For this review, take the finished solid that the model builds, in its own axes (mm). A direction names the side the tool comes from. Round coordinates to 2 decimals unless told otherwise and drop trailing zeros. Order: outer loops, then holes, each group sorted by start corner. A loop starts at its lowest first (then second) coordinate and runs counter-clockwise, first axis right, second up. Notation, with made-up numbers: (80.25, 17) - (135.25, 17) arc R14 cw to (135.25, 41) - close; hole circle Ø3 at (-21, 44.25). An arc over 180 degrees is marked (long way). One line per question, with ' | ' between items.
```python
from build123d import *

# Parameters (mm, degrees)
F0_R     = 15.875
F1_DEPTH = 19.05
F2_R     = 1.27
F3_R     = 6.35
F4_DEPTH = 25.4
F5_R     = 3.175
F6_DEPTH = 12.7


with BuildPart() as f1:
    # F0 (on Front) → F1 (new body)
    with BuildSketch(Plane.XZ):
        Circle(F0_R)
    extrude(amount=-F1_DEPTH)

    # F2
    f2_edges = [f1.edges().sort_by_distance(p)[0] for p in [
        (-15.875, 19.05, 0),
        (-15.875, 0, 0),
    ]]
    fillet(f2_edges, radius=F2_R)

    # F3 (on face) → F4 (join)
    with BuildSketch(Plane(origin=(0, 19.05, 0), x_dir=(-1, 0, 0), z_dir=(0, 1, 0))):
        Circle(F3_R)
    extrude(amount=F4_DEPTH)

    # F5 (on Top) → F6 (cut, symmetric)
    with BuildSketch(Plane.XY):
        with Locations((0, 31.75)):
            Circle(F5_R)
    extrude(amount=F6_DEPTH, both=True, mode=Mode.SUBTRACT)


solid = f1.part
```
(1) We need section B-B on z = 0. State the section outline as (x, y) points (3 decimals), plus the area to 3 significant figures.
Output values:
outline: (-15.875, 1.27) arc R1.27 ccw to (-14.605, 0) - (14.605, 0) arc R1.27 ccw to (15.875, 1.27) - (15.875, 17.78) arc R1.27 ccw to (14.605, 19.05) - (6.35, 19.05) - (6.35, 44.45) - (-6.35, 44.45) - (-6.35, 19.05) - (-14.605, 19.05) arc R1.27 ccw to (-15.875, 17.78) - close; hole circle Ø6.35 at (0, 31.75) | area: 894 mm^2
(2) For probe 1 along Y at (x, z) = (0, -2.75) (3 decimals); probe 2 along X at (y, z) = (31.75, -0.25) (3 decimals); probe 3 along X at (y, z) = (37.5, 5.5), list the stretches that pass through material, from the lowest coordinate up. Write a range as [from, to].
Output values:
probe 1: [0, 28.575], [34.925, 44.45] | probe 2: [-6.345, -3.175], [3.175, 6.345] | probe 3: [-3.17, 3.17]
(3) Insertion check: pin 1 (10 mm diameter, centred on x = -9, y = 11, fed in from +Z); pin 2 (4 mm diameter, centred on x = -9, y = 20.5, fed in from +Z) (3 decimals); pin 3 (4 mm diameter, centred on x = 0, y = 31.75, fed in from +Z); pin 4 (1 mm diameter, centred on y = 6, z = 6, fed in from +X). Each pin has a flat end and moves straight along its axis. Give the tip position at first contact, or say it passes through.
Output values:
pin 1: z = 15.36 | pin 2: z = 13.175 | pin 3: through | pin 4: x = 14.89
(4) We need section A-A on x = 0. State the section outline as (y, z) points (3 decimals), plus the area to 3 significant figures.
Output values:
outline: (0, -14.605) arc R1.27 ccw to (1.27, -15.875) - (17.78, -15.875) arc R1.27 ccw to (19.05, -14.605) - (19.05, -6.35) - (28.575, -6.35) - (28.575, 6.35) - (19.05, 6.35) - (19.05, 14.605) arc R1.27 ccw to (17.78, 15.875) - (1.27, 15.875) arc R1.27 ccw to (0, 14.605) - close; (34.925, -6.35) - (44.45, -6.35) - (44.45, 6.35) - (34.925, 6.35) - close | area: 845 mm^2
(5) We need section D-D on y = 25. State the section outline as (x, z) points.
Output values:
outline: circle Ø12.7 at (0, 0)
(6) For faces 1 (the cylindrical face through (-5.866, 31.572, -2.432)), 2 (the flat face through (0, 44.45, 0)), list the 3-axis set-ups (+Z, -Z, +X, -X, +Y, -Y) from which the entire face can be reached by the end or side of a thin tool; tool diameter is ignored.
Output values:
face 1: +Y | face 2: +Z, -Z, +X, -X, +Y
(7) We need section C-C on y = 33.5. State the section outline as (x, z) points.
Output values:
outline: (-2.65, -5.77) - (-2.65, 5.77) arc R6.35 ccw to start; (2.65, -5.77) arc R6.35 ccw to (2.65, 5.77) - close
(8) Mouldability with a two-part tool opening along X and no side actions: class faces 3 (the flat face through (0, 0, 0)), 4 (the cylindrical face through (-3.441, 9.409, -15.497)), 5 (the cylindrical face through (2.93, 30.53, 0.09)) as released by +X, released by -X, zero draft, split by the parting line, or undercut.
Output values:
face 3: zero draft | face 4: split by the parting line | face 5: undercut
